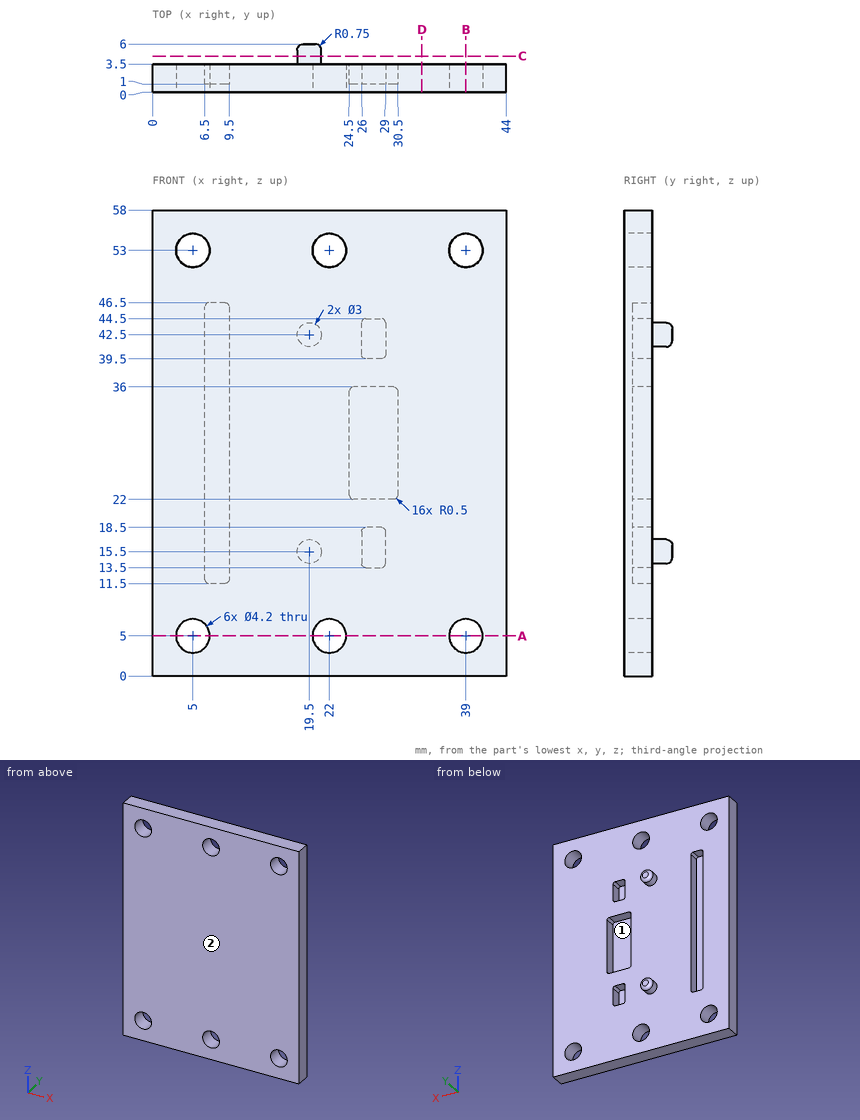
Print and shaded views of the part. All mm, measured from the part's lowest x, y and z. Give positions to 0.01 mm unless a question says otherwise; leave off trailing zeros. Loops run counter-clockwise (first coordinate to the right, second up) from the corner with the lowest first, then second, coordinate; pieces in that order, holes last. Notation, with made-up numbers: (61, -35.5) - (102, -35.5) arc R13 cw to (102, -13.5) - close; hole circle Ø9 at (75, -18). An arc over 180 degrees is marked (long way). One line per item, written item: value. Start each with the question number.
1. Pin check, flat tips, straight feed: pin 1 (3 mm diameter, centred on y = 2, z = 27, fed in from -X); pin 2 (2 mm diameter, centred on x = 18.5, z = 36.5, fed in from +Y); pin 3 (0.9 mm diameter, centred on x = 8.5, z = 31.5, fed in from +Y). Stop position of each tip, or through.
2. Slice it at A-A (z = 5). List the corners of the cut face in (x, y), plus the area to 3 significant figures.
3. Slice it at C-C (y = 4.5). List the corners of the cut face in (x, z).
4. Pull direction X, two halves, no side cores. Call the marked faces 1 and 2: pulls with the +X half, pulls with the -X half, needs draft (parallel to the pull), parting line crosses it, or undercut.
5. Probe L1, parallel to Z at x = 5, y = 1.7; L2, parallel to X at y = 2.5, z = 53; L3, parallel to X at y = 1.3, z = 12.5. List the from-to ranges inside material, lowest first. Write a range as from..to.
6. Slice it at D-D (x = 33.5). List the corners of the cut face in (y, z), plus the area to 3 significant figures.
7. Slice it at B-B (x = 39). List the corners of the cut face in (y, z), plus the area to 3 significant figures.
Solution:
1. pin 1: stops at x = 0
1. pin 2: stops at y = 3.5
1. pin 3: stops at y = 1
2. outline: (0, 0) - (2.9, 0) - (2.9, 3.5) - (0, 3.5) - close; (7.1, 0) - (19.9, 0) - (19.9, 3.5) - (7.1, 3.5) - close; (24.1, 0) - (36.9, 0) - (36.9, 3.5) - (24.1, 3.5) - close; (41.1, 0) - (44, 0) - (44, 3.5) - (41.1, 3.5) - close
2. area: 110 mm^2
3. outline: circle Ø3 at (19.5, 15.5); circle Ø3 at (19.5, 42.5)
4. face 1: undercut
4. face 2: needs draft
5. L1: z = 0..2.9, 7.1..50.9, 55.1..58
5. L2: x = 0..2.9, 7.1..19.9, 24.1..36.9, 41.1..44
5. L3: x = 0..6.5, 9.5..44
6. outline: (0, 0) - (3.5, 0) - (3.5, 58) - (0, 58) - close
6. area: 203 mm^2
7. outline: (0, 0) - (3.5, 0) - (3.5, 2.9) - (0, 2.9) - close; (0, 7.1) - (3.5, 7.1) - (3.5, 50.9) - (0, 50.9) - close; (0, 55.1) - (3.5, 55.1) - (3.5, 58) - (0, 58) - close
7. area: 174 mm^2
